Read the model definition and answer for the solid it produces. Units are mm, in the model's axes. A direction names the side the tool comes from. Round coordinates to 2 decimals unless told otherwise and drop trailing zeros. Write each loop counter-clockwise with the first axis right and the second up, starting at its lowest first coordinate (ties: lowest second). Pieces come first, ordered by that corner, then holes. Notation, with made-up numbers: (-28, 69) - (6, 69) arc R25 ccw to (6, 100) - close; hole circle Ø4 at (-0.75, 66.5). An arc over 180 degrees is marked (long way). Answer as CSV lines item,"result". Start each with the question number.
1) Find section B-B on z = 424. Determine the outline of the cut face in (x, y) (3 decimals).
2) For a pull along Z with two mould halves and no side action, classify faces 1 (the cylindrical face through (-11.09, -1.852, 204.652)), 2 (the flat face through (-10, -2, 0)), 3 (the cylindrical face through (-11.09, -3.08, 676.66)), 4 (the flat face through (9.525, 0, 376)) as +Z half, -Z half, draft (parallel to the pull), parting line (faces both ways), or undercut.
3) Find section A-A on y = 0. Determine the outline of the cut face in (x, z) (3 decimals).
4) This flat-tipped pin is pushed along its axis until it touches: pin 1 (3.5 mm diameter, centred on x = -2.54, z = 264.16, fed in from -Y) (3 decimals). Where does it stop, or does it pass through?
5) Consider line 1 along X through (y, z) = (-24.2, 264.16); line 2 along Z through (x, y) = (10.55, 0); line 3 along X through (y, z) = (-4, 437.5) (3 decimals). Determine where each line is inside the solid, lowest interval first.
6) Which of the six approach directions +Z, -Z, +X, -X, +Y, -Y give full straight-line access (tool end or side, diameter ignored) to faces 5 (the flat face through (0, 22.225, 376)), 6 (the flat face through (12.7, 0, 376))?
from build123d import *

# Parameters (mm, degrees)
SKETCH1_W           = 25.4
SKETCH1_H           = 50.8
SKETCH1_W_2         = 19.05
SKETCH1_H_2         = 44.45
BOSS_EXTRUDE1_DEPTH = 762
CUT_EXTRUDE1_REACH  = 764.846
SKETCH4_R           = 14.224
SKETCH5_R           = 2.0955
CUT_EXTRUDE2_DEPTH  = 3.175
CUT_EXTRUDE3_REACH  = 764.846
SKETCH7_R           = 2.0955


with BuildPart() as part:
    # Sketch1 → Boss-Extrude1 (new body)
    with BuildSketch(Plane.XY):
        Rectangle(SKETCH1_W, SKETCH1_H)
        Rectangle(SKETCH1_W_2, SKETCH1_H_2, mode=Mode.SUBTRACT)
    extrude(amount=BOSS_EXTRUDE1_DEPTH)

    # Cut-Extrude1: up to this face of the body (flat: up to its plane)
    cut_extrude1_end = Plane(part.part.faces().sort_by_distance((-12.7, 0, 381))[0])
    # Sketch4 → Cut-Extrude1 (cut, up to the picked face)
    with BuildSketch(Plane(origin=(12.7, 0, 0), x_dir=(0, 0, -1), z_dir=(1, 0, 0)), mode=Mode.PRIVATE) as cut_extrude1_sk1:
        with Locations(Location((-690.548048411, 0, 0), (0, 0, 90))):
            Circle(SKETCH4_R)
    cut_extrude1_tool1 = split(extrude(cut_extrude1_sk1.sketch, amount=-CUT_EXTRUDE1_REACH, mode=Mode.PRIVATE), bisect_by=cut_extrude1_end, keep=Keep.BOTH, mode=Mode.PRIVATE)
    # Sketch4 → Cut-Extrude1 (cut, up to the picked face)
    with BuildSketch(Plane(origin=(12.7, 0, 0), x_dir=(0, 0, -1), z_dir=(1, 0, 0)), mode=Mode.PRIVATE) as cut_extrude1_sk2:
        with Locations(Location((-190.549048411, 0, 0), (0, 0, 90))):
            Circle(SKETCH4_R)
    cut_extrude1_tool2 = split(extrude(cut_extrude1_sk2.sketch, amount=-CUT_EXTRUDE1_REACH, mode=Mode.PRIVATE), bisect_by=cut_extrude1_end, keep=Keep.BOTH, mode=Mode.PRIVATE)
    add(cut_extrude1_tool1.solids().sort_by(Axis((12.7, 0, 690.548048), (-1, 0, 0)))[0], mode=Mode.SUBTRACT)
    add(cut_extrude1_tool2.solids().sort_by(Axis((12.7, 0, 190.549048), (-1, 0, 0)))[0], mode=Mode.SUBTRACT)

    # Sketch5 → Cut-Extrude2 (cut)
    with BuildSketch(Plane.XZ.offset(25.4)):
        with Locations(Location((2.54, 264.16, 0), (0, 0, 270))):
            Circle(SKETCH5_R)
        with Locations(Location((2.54, 289.56, 0), (0, 0, 270))):
            Circle(SKETCH5_R)
        with Locations(Location((2.54, 314.96, 0), (0, 0, 270))):
            Circle(SKETCH5_R)
        with Locations(Location((-2.54, 264.16, 0), (0, 0, 180))):
            Circle(SKETCH5_R)
        with Locations(Location((-2.54, 289.56, 0), (0, 0, 180))):
            Circle(SKETCH5_R)
        with Locations(Location((-2.54, 314.96, 0), (0, 0, 180))):
            Circle(SKETCH5_R)
    extrude(amount=-CUT_EXTRUDE2_DEPTH, mode=Mode.SUBTRACT)

    # Cut-Extrude3: up to this face of the body (flat: up to its plane)
    cut_extrude3_end = Plane(part.part.faces().sort_by_distance((-12.7, 0, 378.978016644))[0])
    # Sketch7 → Cut-Extrude3 (cut, up to the picked face)
    with BuildSketch(Plane(origin=(12.7, 0, 0), x_dir=(0, 0, -1), z_dir=(1, 0, 0)), mode=Mode.PRIVATE) as cut_extrude3_sk1:
        with Locations(Location((-259.08, -15.24, 0), (0, 0, 90))):
            Circle(SKETCH7_R)
    cut_extrude3_tool1 = split(extrude(cut_extrude3_sk1.sketch, amount=-CUT_EXTRUDE3_REACH, mode=Mode.PRIVATE), bisect_by=cut_extrude3_end, keep=Keep.BOTH, mode=Mode.PRIVATE)
    # Sketch7 → Cut-Extrude3 (cut, up to the picked face)
    with BuildSketch(Plane(origin=(12.7, 0, 0), x_dir=(0, 0, -1), z_dir=(1, 0, 0)), mode=Mode.PRIVATE) as cut_extrude3_sk2:
        with Locations(Location((-284.48, -15.24, 0), (0, 0, 90))):
            Circle(SKETCH7_R)
    cut_extrude3_tool2 = split(extrude(cut_extrude3_sk2.sketch, amount=-CUT_EXTRUDE3_REACH, mode=Mode.PRIVATE), bisect_by=cut_extrude3_end, keep=Keep.BOTH, mode=Mode.PRIVATE)
    # Sketch7 → Cut-Extrude3 (cut, up to the picked face)
    with BuildSketch(Plane(origin=(12.7, 0, 0), x_dir=(0, 0, -1), z_dir=(1, 0, 0)), mode=Mode.PRIVATE) as cut_extrude3_sk3:
        with Locations(Location((-309.88, -15.24, 0), (0, 0, 90))):
            Circle(SKETCH7_R)
    cut_extrude3_tool3 = split(extrude(cut_extrude3_sk3.sketch, amount=-CUT_EXTRUDE3_REACH, mode=Mode.PRIVATE), bisect_by=cut_extrude3_end, keep=Keep.BOTH, mode=Mode.PRIVATE)
    # Sketch7 → Cut-Extrude3 (cut, up to the picked face)
    with BuildSketch(Plane(origin=(12.7, 0, 0), x_dir=(0, 0, -1), z_dir=(1, 0, 0)), mode=Mode.PRIVATE) as cut_extrude3_sk4:
        with Locations(Location((-87.63, -15.24, 0), (0, 0, 90))):
            Circle(SKETCH7_R)
    cut_extrude3_tool4 = split(extrude(cut_extrude3_sk4.sketch, amount=-CUT_EXTRUDE3_REACH, mode=Mode.PRIVATE), bisect_by=cut_extrude3_end, keep=Keep.BOTH, mode=Mode.PRIVATE)
    # Sketch7 → Cut-Extrude3 (cut, up to the picked face)
    with BuildSketch(Plane(origin=(12.7, 0, 0), x_dir=(0, 0, -1), z_dir=(1, 0, 0)), mode=Mode.PRIVATE) as cut_extrude3_sk5:
        with Locations(Location((-62.23, -15.24, 0), (0, 0, 90))):
            Circle(SKETCH7_R)
    cut_extrude3_tool5 = split(extrude(cut_extrude3_sk5.sketch, amount=-CUT_EXTRUDE3_REACH, mode=Mode.PRIVATE), bisect_by=cut_extrude3_end, keep=Keep.BOTH, mode=Mode.PRIVATE)
    # Sketch7 → Cut-Extrude3 (cut, up to the picked face)
    with BuildSketch(Plane(origin=(12.7, 0, 0), x_dir=(0, 0, -1), z_dir=(1, 0, 0)), mode=Mode.PRIVATE) as cut_extrude3_sk6:
        with Locations(Location((-113.03, -15.24, 0), (0, 0, 90))):
            Circle(SKETCH7_R)
    cut_extrude3_tool6 = split(extrude(cut_extrude3_sk6.sketch, amount=-CUT_EXTRUDE3_REACH, mode=Mode.PRIVATE), bisect_by=cut_extrude3_end, keep=Keep.BOTH, mode=Mode.PRIVATE)
    add(cut_extrude3_tool1.solids().sort_by(Axis((12.7, -15.24, 259.08), (-1, 0, 0)))[0], mode=Mode.SUBTRACT)
    add(cut_extrude3_tool2.solids().sort_by(Axis((12.7, -15.24, 284.48), (-1, 0, 0)))[0], mode=Mode.SUBTRACT)
    add(cut_extrude3_tool3.solids().sort_by(Axis((12.7, -15.24, 309.88), (-1, 0, 0)))[0], mode=Mode.SUBTRACT)
    add(cut_extrude3_tool4.solids().sort_by(Axis((12.7, -15.24, 87.63), (-1, 0, 0)))[0], mode=Mode.SUBTRACT)
    add(cut_extrude3_tool5.solids().sort_by(Axis((12.7, -15.24, 62.23), (-1, 0, 0)))[0], mode=Mode.SUBTRACT)
    add(cut_extrude3_tool6.solids().sort_by(Axis((12.7, -15.24, 113.03), (-1, 0, 0)))[0], mode=Mode.SUBTRACT)


solid = part.part
Check values:
1,outline,"(-12.7, -25.4) - (12.7, -25.4) - (12.7, 25.4) - (-12.7, 25.4) - close; hole (-9.525, -22.225) - (9.525, -22.225) - (9.525, 22.225) - (-9.525, 22.225) - close"
2,face 1,"undercut"
2,face 2,"-Z half"
2,face 3,"undercut"
2,face 4,"draft"
3,outline,"(-12.7, 0) - (-9.525, 0) - (-9.525, 176.325) - (-12.7, 176.325) - close; (-12.7, 204.773) - (-9.525, 204.773) - (-9.525, 676.324) - (-12.7, 676.324) - close; (-12.7, 704.772) - (-9.525, 704.772) - (-9.525, 762) - (-12.7, 762) - close; (9.525, 0) - (12.7, 0) - (12.7, 176.325) - (9.525, 176.325) - close; (9.525, 204.773) - (12.7, 204.773) - (12.7, 676.324) - (9.525, 676.324) - close; (9.525, 704.772) - (12.7, 704.772) - (12.7, 762) - (9.525, 762) - close"
4,pin 1,"stops at y = 22.225"
5,line 1,"x = -12.7 to -4.64, -0.44 to 0.44, 4.64 to 12.7"
5,line 2,"z = 0 to 176.33, 204.77 to 676.32, 704.77 to 762"
5,line 3,"x = -12.7 to -9.525, 9.525 to 12.7"
6,face 5,"+Z, -Z"
6,face 6,"+Z, -Z, +X, +Y, -Y"
